Geometry check sheet. Reference: the model listing, model coordinates, mm. A direction names the side the tool comes from. Give positions to 0.01 mm unless a question says otherwise; leave off trailing zeros. Loops run counter-clockwise (first coordinate to the right, second up) from the corner with the lowest first, then second, coordinate; pieces in that order, holes last. Notation, with made-up numbers: (77.5, 44.25) -> (127.5, 44.25) arc R21 cw to (127.5, 62.25) -> close; hole circle Ø10 at (70.25, -5). An arc over 180 degrees is marked (long way). Write item = value, one per line.
```python
from build123d import *

# Parameters (mm, degrees)
BOSS_EXTRUDE1_DEPTH = 20
SKETCH2_W           = 3
SKETCH2_H           = 6
FILLET1_R           = 1


with BuildPart() as part:
    # Sketch1 → Boss-Extrude1 (new body)
    with BuildSketch(Plane(origin=(0, 0, 0), x_dir=(1, 0, 0), z_dir=(0, 1, 0))):
        with BuildLine():
            Line((-13.097063825, 30.526339541), (-13.097063825, 9.190588619))
            ThreePointArc((-13.097063825, 9.190588619), (0, 16), (13.097063825, 9.190588619))
            Line((13.097063825, 9.190588619), (13.097063825, 30.526339541))
            ThreePointArc((13.097063825, 30.526339541), (0, 29), (-13.097063825, 30.526339541))
        make_face()
    extrude(amount=BOSS_EXTRUDE1_DEPTH)

    # Sketch2 → Cut-Revolve1 (revolve, cut)
    with BuildSketch(Plane(origin=(0, 0, 0), x_dir=(0, 0, -1), z_dir=(1, 0, 0))):
        with Locations((22.074416819, 10)):
            Rectangle(SKETCH2_W, SKETCH2_H)
    revolve(axis=Axis((0, 0, 0), (0, 1, 0)), mode=Mode.SUBTRACT)

    # Fillet1
    fillet1_edges = [part.edges().sort_by_distance(p)[0] for p in [
        (0, 20, -16),
        (13.097063825, 13, -17.734452708),
        (13.097063825, 10, -19.601531765),
        (13.097063825, 7, -17.734452708),
        (13.097063825, 10, -15.867373652),
        (13.097063825, 20, -19.85846408),
        (-13.097063825, 10, -15.867373652),
        (-13.097063825, 7, -17.734452708),
        (-13.097063825, 10, -19.601531765),
        (-13.097063825, 13, -17.734452708),
        (0, 20, -29),
        (13.097063825, 0, -19.85846408),
        (0, 0, -16),
        (-13.097063825, 0, -19.85846408),
        (0, 0, -29),
        (13.097063825, 10, -30.526339541),
        (13.097063825, 10, -9.190588619),
        (-13.097063825, 10, -9.190588619),
        (-13.097063825, 10, -30.526339541),
        (-13.097063825, 20, -19.85846408),
    ]]
    fillet(fillet1_edges, radius=FILLET1_R)


solid = part.part
```
Item 1: Section check C-C, the plane y = 5. Record the cut outline in (x, z), plus the area to 3 significant figures.
Answer:
outline = (-13.1, -29.28) arc R1 ccw to (-11.89, -30.25) arc R56.95 cw to (11.89, -30.25) arc R1 ccw to (13.1, -29.28) -> (13.1, -11.94) arc R1 ccw to (11.39, -11.24) arc R16 cw to (-11.39, -11.24) arc R1 ccw to (-13.1, -11.94) -> close
area = 403 mm^2
Item 2: Draft check along X on faces 1 (the cylindrical face through (-12.81, 6.7, -18.43)), 2 (the cylindrical face through (12.81, 6.7, -18.35)), 3 (the flat face through (0, 7, -21)). Enter one of: +X half, -X half, draft (parallel to the pull), parting line (faces both ways), or undercut.
Answer:
face_1 = -X half
face_2 = +X half
face_3 = undercut
Item 3: Gauge pin test, flat ends, axial feed: pin 1 (2 mm diameter, centred on x = -9.5, y = 16, fed in from +Z); pin 2 (8 mm diameter, centred on x = 2, y = 4.5, fed in from +Z); pin 3 (2 mm diameter, centred on x = -6.5, y = 7, fed in from +Z). Record the tip position at first contact, or that the pin passes through.
Answer:
pin_1 = -12.07
pin_2 = -14.83
pin_3 = -14.13
Item 4: Thickness scan on L1, parallel to Y at x = -0.25, z = -21; L2, parallel to Z at x = 0, y = 15.75; L3, parallel to Z at x = -7.25, y = 8.75. Record the ranges inside material, lowest first. Write a range as [from, to].
Answer:
L1 = [0, 7], [13, 20]
L2 = [-29, -16]
L3 = [-29.46, -22.43], [-19.25, -14.26]
Item 5: Section check A-A, the plane y = 8. Record the cut outline in (x, z), plus the area to 3 significant figures.
Answer:
outline = (-13.1, -29.28) arc R1 ccw to (-11.89, -30.25) arc R56.95 cw to (11.89, -30.25) arc R1 ccw to (13.1, -29.28) -> (13.1, -21.39) arc R1 ccw to (11.6, -20.52) arc R23.57 cw to (-11.6, -20.52) arc R1 ccw to (-13.1, -21.39) -> close; (-13.1, -15.39) arc R1 ccw to (-12.72, -16.18) arc R20.57 ccw to (12.72, -16.18) arc R1 ccw to (13.1, -15.39) -> (13.1, -11.94) arc R1 ccw to (11.39, -11.24) arc R16 cw to (-11.39, -11.24) arc R1 ccw to (-13.1, -11.94) -> close
area = 318 mm^2
Item 6: Section check B-B, the plane z = -18.5. Record the cut outline in (x, y), plus the area to 3 significant figures.
Answer:
outline = (-13.1, 1) arc R1 ccw to (-12.1, 0) -> (12.1, 0) arc R1 ccw to (13.1, 1) -> (13.1, 6) arc R1 ccw to (12.1, 7) -> (9, 7) -> (9, 13) -> (12.1, 13) arc R1 ccw to (13.1, 14) -> (13.1, 19) arc R1 ccw to (12.1, 20) -> (-12.1, 20) arc R1 ccw to (-13.1, 19) -> (-13.1, 14) arc R1 ccw to (-12.1, 13) -> (-9, 13) -> (-9, 7) -> (-12.1, 7) arc R1 ccw to (-13.1, 6) -> close
area = 473 mm^2
Item 7: Tool access check on faces 4 (the cylindrical face through (0.17, 10.042, -23.574)), 5 (the cylindrical face through (-12.81, 13.3, -18.43)), 6 (the cylindrical face through (-12.492, 10.126, -11.025)). Record the directions out of +Z, -Z, +X, -X, +Y, -Y that give a thin tool (end or side, any length) a straight path to the whole face; none if there is none.
Answer:
face_4 = none
face_5 = -X
face_6 = +Z, +Y, -Y
